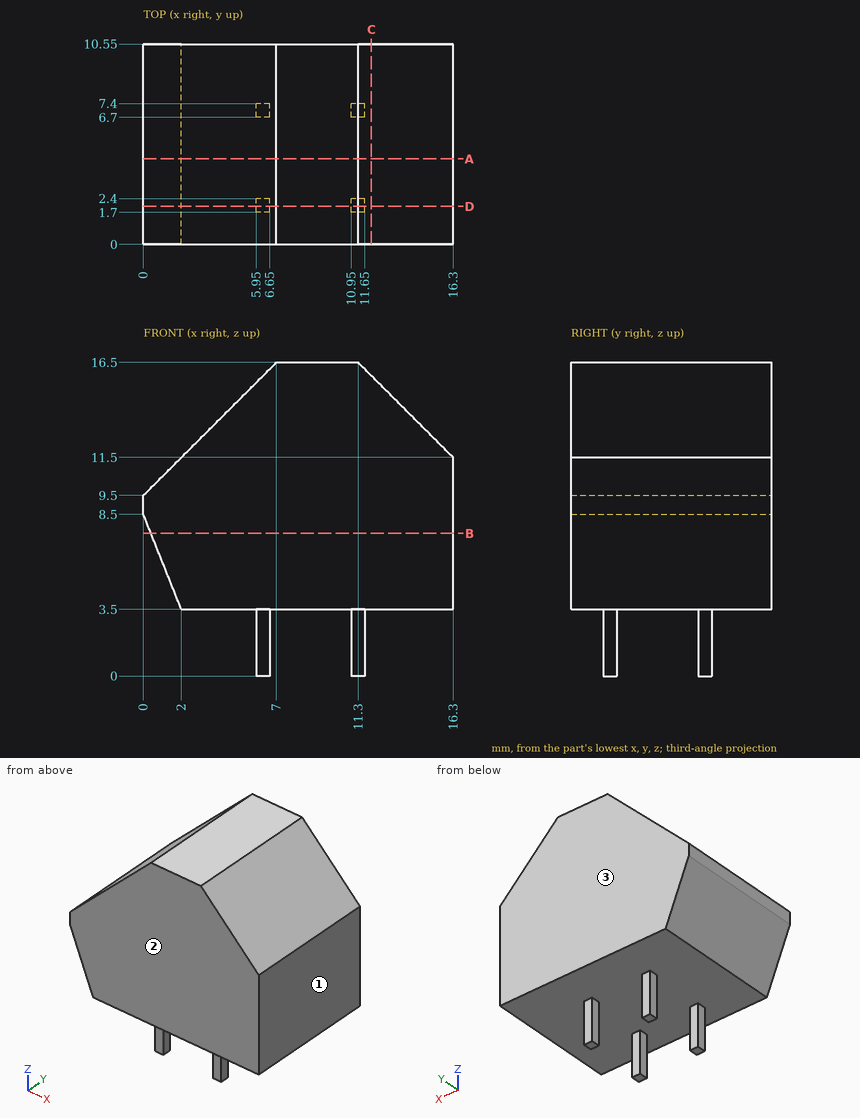
Could you check a few things on this drawing? It's one solid part, dimensions in mm from its lowest x, y, z. Round coordinates to 2 decimals unless told otherwise and drop trailing zeros. Order: outer loops, then holes, each group sorted by start corner. A loop starts at its lowest first (then second) coordinate and runs counter-clockwise, first axis right, second up. Notation, with made-up numbers: (68.25, 52) -> (75.25, 52) arc R7 ccw to (75.25, 62) -> close; hole circle Ø9 at (-16, -28.5). An arc over 180 degrees is marked (long way). One line per question, with ' | ' between items.
Q1. If I drill on line 1 (Z direction, x = 7.75, y = 10); line 2 (Z direction, x = 3.75, y = 2); line 3 (X direction, y = 2, z = 8), over which ranges is the centre line in solid material (lowest first)? Write a range as from..to.
Computed values:
line 1: 3.5..16.5 | line 2: 3.5..13.25 | line 3: 0.2..16.3
Q2. If we section it at A-A on y = 4.5: Write out the boundary of the cut face in (x, z), plus the area to 3 significant figures.
Computed values:
outline: (0, 8.5) -> (2, 3.5) -> (16.3, 3.5) -> (16.3, 11.5) -> (11.3, 16.5) -> (7, 16.5) -> (0, 9.5) -> close | area: 170 mm²
Q3. If we section it at D-D on y = 2: Write out the boundary of the cut face in (x, z), plus the area to 3 significant figures.
Computed values:
outline: (0, 8.5) -> (2, 3.5) -> (5.95, 3.5) -> (5.95, 0) -> (6.65, 0) -> (6.65, 3.5) -> (10.95, 3.5) -> (10.95, 0) -> (11.65, 0) -> (11.65, 3.5) -> (16.3, 3.5) -> (16.3, 11.5) -> (11.3, 16.5) -> (7, 16.5) -> (0, 9.5) -> close | area: 175 mm²
Q4. If we section it at C-C on x = 12: Write out the boundary of the cut face in (y, z), plus the area to 3 significant figures.
Computed values:
outline: (0, 3.5) -> (10.55, 3.5) -> (10.55, 15.8) -> (0, 15.8) -> close | area: 130 mm²
Q5. We'd pull the mould along Y, two halves only. Please class the marked faces 1, 2 and 3: released by +Y, released by -Y, zero draft, split by the parting line, or undercut.
Computed values:
face 1: zero draft | face 2: released by -Y | face 3: released by +Y
Q6. I'm going to push flat-ended pins straight in: pin 1 (0.6 mm diameter, centred on x = 6.5, z = 2, fed in from +Y); pin 2 (0.8 mm diameter, centred on x = 6, z = 1.5, fed in from -Y); pin 3 (0.8 mm diameter, centred on y = 2, z = 1.5, fed in from -X). Where does each tip first touch, or does it pass through?
Computed values:
pin 1: y = 7.4 | pin 2: y = 1.7 | pin 3: x = 5.95
Q7. If we section it at B-B on z = 7.5: Write out the boundary of the cut face in (x, y).
Computed values:
outline: (0.4, 0) -> (16.3, 0) -> (16.3, 10.55) -> (0.4, 10.55) -> close
